```python
from build123d import *

# Parameters (mm, degrees)
SKETCH1_W           = 40
SKETCH1_H           = 8
SKETCH1_R           = 2.2
BOSS_EXTRUDE1_DEPTH = 3


with BuildPart() as part:
    # Sketch1 → Boss-Extrude1 (new body)
    with BuildSketch(Plane.XY):
        with Locations((0.002263133, 1)):
            Rectangle(SKETCH1_W, SKETCH1_H)
        with Locations((0.002263133, 1)):
            Circle(SKETCH1_R, mode=Mode.SUBTRACT)
        with BuildLine():
            ThreePointArc((-11.98520546, 1.25), (-11.997736867, 1), (-11.98520546, 0.75))
            ThreePointArc((-11.98520546, 0.75), (-6.997736867, 1), (-11.98520546, 1.25))
        make_face(mode=Mode.SUBTRACT)
        with BuildLine():
            ThreePointArc((11.98520546, 1.25), (6.997736867, 1), (11.98520546, 0.75))
            ThreePointArc((11.98520546, 0.75), (11.997736867, 1), (11.98520546, 1.25))
        make_face(mode=Mode.SUBTRACT)
    extrude(amount=BOSS_EXTRUDE1_DEPTH)


solid = part.part
```
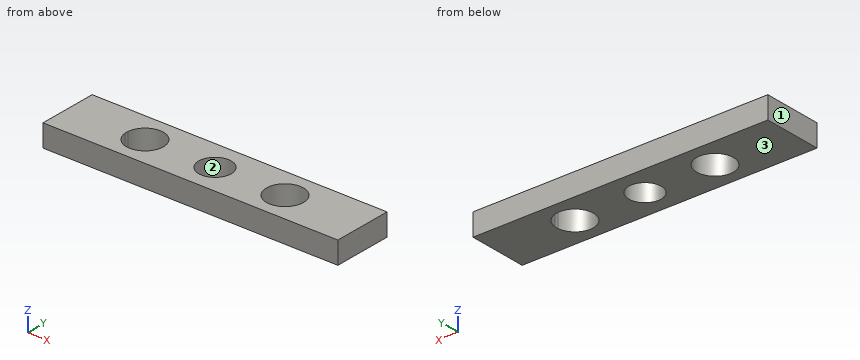
Work out the finished part from the listing and answer in its coordinate system (mm). Face numbers are marked on the shaded views. Give positions to 0.01 mm unless a question says otherwise; leave off trailing zeros. Write each loop counter-clockwise with the first axis right and the second up, starting at its lowest first coordinate (ties: lowest second). Pieces come first, ordered by that corner, then holes. Notation, with made-up numbers: (64, 87) -> (112, 87) arc R32 ccw to (112, 117) -> close; hole circle Ø2 at (26, 82.5). An arc over 180 degrees is marked (long way). Write item = value, one per line.
Q1. Consider line 1 along Y through (x, z) = (-9.5, 1.7); line 2 along X through (y, z) = (2, 0.35); line 3 along X through (y, z) = (1.75, 0.25). Determine where each line is inside the solid, lowest interval first.
Computed values:
line_1 = -3 to -1.5, 3.5 to 5
line_2 = -20 to -11.79, -7.21 to -1.96, 1.96 to 7.21, 11.79 to 20
line_3 = -20 to -11.88, -7.11 to -2.07, 2.07 to 7.11, 11.88 to 20
Q2. Section C-C on y = 2 is taken. Determine the outline of the cut face in (x, z), and give its area (3 significant figures).
Computed values:
outline = (-20, 0) -> (-11.79, 0) -> (-11.79, 3) -> (-20, 3) -> close; (-7.21, 0) -> (-1.96, 0) -> (-1.96, 3) -> (-7.21, 3) -> close; (1.96, 0) -> (7.21, 0) -> (7.21, 3) -> (1.96, 3) -> close; (11.79, 0) -> (20, 0) -> (20, 3) -> (11.79, 3) -> close
area = 80.7 mm^2
Q3. Section B-B on z = 1 is taken. Determine the outline of the cut face in (x, y).
Computed values:
outline = (-20, -3) -> (20, -3) -> (20, 5) -> (-20, 5) -> close; hole circle Ø5 at (-9.5, 1); hole circle Ø4.4 at (0, 1); hole circle Ø5 at (9.5, 1)
Q4. Section A-A on x = -8 is taken. Determine the outline of the cut face in (y, z), and give its area (3 significant figures).
Computed values:
outline = (-3, 0) -> (-1, 0) -> (-1, 3) -> (-3, 3) -> close; (3, 0) -> (5, 0) -> (5, 3) -> (3, 3) -> close
area = 12.0 mm^2
Q5. For a pull along X with two mould halves and no side action, classify the marked faces 1, 2 and 3 as pulls with the +X half, pulls with the -X half, needs draft (parallel to the pull), parting line crosses it, or undercut.
Computed values:
face_1 = pulls with the -X half
face_2 = undercut
face_3 = needs draft
Q6. Section D-D on x = 1.5 is taken. Determine the outline of the cut face in (y, z).
Computed values:
outline = (-3, 0) -> (-0.61, 0) -> (-0.61, 3) -> (-3, 3) -> close; (2.61, 0) -> (5, 0) -> (5, 3) -> (2.61, 3) -> close
